Verification items for the finished model (mm, model axes). A direction names the side the tool comes from. Round coordinates to 2 decimals unless told otherwise and drop trailing zeros. Loops run counter-clockwise (first coordinate to the right, second up) from the corner with the lowest first, then second, coordinate; pieces in that order, holes last. Notation, with made-up numbers: M -11.75,-21 L 8.25,-21 A26 ccw 8.25,-1 Z; hole C 81.5,16 d8. An arc over 180 degrees is marked long. Answer as CSV lines item,"result".
```python
from build123d import *

# Parameters (mm, degrees)
PAD005_DEPTH            = 32
SKETCH013_W             = 337.5
SKETCH013_H             = 19
POCKET007_DEPTH         = 9.5
SKETCH014_W             = 337.5
SKETCH014_H             = 4
POCKET008_DEPTH         = 4
SKETCH015_W             = 337.5
SKETCH015_H             = 32
POCKET009_DEPTH         = 6
BODY004_PLACEMENT_ANGLE = 90


with BuildPart() as part:
    # Sketch012 → Pad005 (new body)
    with BuildSketch(Plane.XY):
        with BuildLine():
            Line((18, 65), (319.5, 65))
            ThreePointArc((337.5, 47), (332.227922, 59.727922), (319.5, 65))
            Line((337.5, 47), (337.5, 0))
            Line((337.5, 0), (0, 0))
            Line((0, 0), (0, 47))
            ThreePointArc((18, 65), (5.272078, 59.727922), (0, 47))
        make_face()
    extrude(amount=PAD005_DEPTH)

    # Sketch013 (on Face8 of Pad005) → Pocket007 (cut)
    with BuildSketch(Plane.XY.offset(32)):
        with Locations((168.75, 35.5)):
            Rectangle(SKETCH013_W, SKETCH013_H)
    extrude(amount=-POCKET007_DEPTH, mode=Mode.SUBTRACT)

    # Sketch014 (on Face4 of Pocket007) → Pocket008 (cut)
    with BuildSketch(Plane.XY.offset(32)):
        with Locations((168.75, 2)):
            Rectangle(SKETCH014_W, SKETCH014_H)
    extrude(amount=-POCKET008_DEPTH, mode=Mode.SUBTRACT)

    # Sketch015 (on Face2 of Pocket008) → Pocket009 (cut)
    with BuildSketch(Plane(origin=(0, 0, 0), x_dir=(1, 0, 0), z_dir=(0, 0, -1))):
        with Locations((168.75, -16)):
            Rectangle(SKETCH015_W, SKETCH015_H)
    extrude(amount=-POCKET009_DEPTH, mode=Mode.SUBTRACT)


with BuildPart() as part_1:
    # Body004 placement: moved
    add(part.part.moved(Location((22.5, 6, 0))).rotate(Axis((22.5, 6, 0), (1, 0, 0)), BODY004_PLACEMENT_ANGLE))


with BuildPart() as part_2:
    # Body006 placement: moved
    add(part_1.part.moved(Location((-382.5, 0, 0))))


solid = part_2.part
```
1) Section check A-A (x = -236). Record the cut outline in (y, z).
Here are the results:
outline,"M -26,4 L -22,4 L -22,0 L 0,0 L 0,32 L 6,32 L 6,65 L -26,65 L -26,45 L -16.5,45 L -16.5,26 L -26,26 Z"
2) Material ranges on probe 1 along Z at (x, y) = (-185, -18); probe 2 along Y at (x, z) = (-128, 20); probe 3 along Z at (x, y) = (-156, 3), recorded low to high.
Here are the results:
probe 1,"z = 0 to 26, 45 to 65"
probe 2,"y = -26 to 0"
probe 3,"z = 32 to 65"
3) Section check C-C (z = 37.5). Record the cut outline in (x, y).
Here are the results:
outline,"M -360,-16.5 L -22.5,-16.5 L -22.5,6 L -360,6 Z"
4) Set-up check for faces 1 (the flat face through (-194, 0, 16)), 2 (the flat face through (-189, 6, 49)), 3 (the flat face through (-194, -16.5, 36)): record each of +Z, -Z, +X, -X, +Y, -Y from which the full face is reachable in a straight line by a thin tool's end or side.
Here are the results:
face 1,"-Z, +X, -X, +Y"
face 2,"+Z, -Z, +X, -X, +Y"
face 3,"+X, -X, -Y"
5) Draft check along Z on faces 4 (the flat face through (-194, -21, 26)), 5 (the cylindrical face through (-27.633, -9.776, 59.587)), 6 (the flat face through (-189, -26, 55)). Enter one of: +Z half, -Z half, draft (parallel to the pull), parting line (faces both ways), or undercut.
Here are the results:
face 4,"undercut"
face 5,"+Z half"
face 6,"draft"
6) Section check B-B (z = 17). Record the cut outline in (x, y), plus the area to 4 significant figures.
Here are the results:
outline,"M -360,-26 L -22.5,-26 L -22.5,0 L -360,0 Z"
area,"8,775 mm^2"
7) Go/stop test with flat-tipped pins: pin 1 (3 mm diameter, centred on x = -160, y = 4, fed in from -Z); pin 2 (1.5 mm diameter, centred on y = -10, z = 51.5, fed in from -X); pin 3 (3 mm diameter, centred on x = -138.5, y = -25, fed in from -Z); pin 4 (21 mm diameter, centred on x = -140.5, z = 34.5, fed in from -Y). Record where each tip stops, or that it passes through.
Here are the results:
pin 1,"stops at z = 32"
pin 2,"stops at x = -359.61"
pin 3,"stops at z = 4"
pin 4,"stops at y = -26"
